Part model, mm, in its own coordinate system. A direction names the side the tool comes from. Coordinates: 2 decimals unless noted, no trailing zeros. Write each loop counter-clockwise with the first axis right and the second up, starting at its lowest first coordinate (ties: lowest second). Pieces come first, ordered by that corner, then holes. Notation, with made-up numbers: M 88,6.5 L 128,6.5 A6 cw 128,15.5 Z; hole C 10.5,-3.5 d3. An arc over 180 degrees is marked long. Use a Markdown table: item, result. Add a question column.
Q1. Slice it at D-D on x = -17.5. Write the cut outline in (y, z), then the cut area to 3 significant figures.
Q2. Slice it at B-B on z = 18.5. Write the cut outline in (x, y).
Q3. Slice it at C-C on y = 1.5. Write the cut outline in (x, z).
Q4. Slice it at A-A on x = -42. Write the cut outline in (y, z), then the cut area to 3 significant figures.
Q5. Wall check: L1, parallel to Z at x = -35.5, y = 9.75; L2, parallel to Z at x = -53.5, y = 1; L3, parallel to X at y = 1.5, z = 12. Give the ranges that are in metal, low to high. Write a range as from..to.
Q6. Tool access for faces 1 (the flat face through (-26, 23.72, 47)), 2 (the flat face through (-15, 3.72, 24)), 3 (the flat face through (-26, 17.72, 45)): list every direction of +Z, -Z, +X, -X, +Y, -Y with a clear straight run to the whole face (end or side of a thin tool).
Q7. Pin check, flat tips, straight feed: pin 1 Ø5.5 at (x, z) = (-25.82, 35.92) entering from -Y; pin 2 Ø0.5 at (x, z) = (-15, 43.5) entering from +Y; pin 3 Ø1 at (x, z) = (-23.5, 9.5) entering from +Y. Stop position of each tip, or through.
Q8. Mould opens along Y. For faces 4 (the flat face through (-44, 22.72, 1)), 5 (the conical face through (-46.144, 12.179, 5.854)), 6 (the flat face through (-26, 17.72, 3)) say: released by +Y, released by -Y, zero draft, split by the parting line, or undercut.
from build123d import *

# Parameters (mm, degrees)
SKETCH_1_W             = 25
SKETCH_1_H             = 25
EXTRUDE_1_DEPTH        = 4
SKETCH_2_W             = 24
SKETCH_2_H             = 24
EXTRUDE_2_DEPTH        = 2
SKETCH_3_R             = 5.625
EXTRUDE_3_DEPTH        = 4
CHAMFER_1_SIZE         = 3
CHAMFER_1_SIZE2        = 0.803847577
EXTRUDE_4_DEPTH        = 2
SKETCH_6_R             = 5
CUT_EXTRUDE_2_DEPTH    = 10
EXTRUDE_6_DEPTH        = 20
SKETCH_9_W             = 19
SKETCH_9_H             = 3
CUT_EXTRUDE_4_DEPTH    = 2
CHAMFER_2_SIZE         = 1
CHAMFER_3_SIZE         = 3.732050808
CHAMFER_3_SIZE_2       = 1
FILLET_1_R             = 13
CHAMFER_4_SIZE         = 1
SKETCH_11_W            = 3
SKETCH_11_H            = 4
EXTRUDE_7_DEPTH        = 16
PATTERN_LINEAR_1_COUNT = 2
PATTERN_LINEAR_1_PITCH = 22
CHAMFER_6_SIZE         = 3
FILLET_2_R             = 1.5
SKETCH_13_W            = 40.293086247
SKETCH_13_H            = 27.591529789
CUT_EXTRUDE_6_DEPTH    = 100
SKETCH_14_R            = 3
CUT_EXTRUDE_7_DEPTH    = 100
CHAMFER_7_SIZE         = 1.5


with BuildPart() as part:
    # Эскиз1 → Бобышка-Вытянуть1 (new body)
    with BuildSketch(Plane.XY):
        with Locations((-26.279531703, 11.219512195)):
            Rectangle(SKETCH_1_W, SKETCH_1_H)
    extrude(amount=EXTRUDE_1_DEPTH)

    # Эскиз2 → Бобышка-Вытянуть2 (add)
    with BuildSketch(Plane(origin=(0, 0, 0), x_dir=(-1, 0, 0), z_dir=(0, 0, -1))):
        with Locations((50.779531703, 10.719512195)):
            Rectangle(SKETCH_2_W, SKETCH_2_H)
    extrude(amount=-EXTRUDE_2_DEPTH)

    # Эскиз3 → Бобышка-Вытянуть3 (add)
    with BuildSketch(Plane.XY.offset(2)):
        with Locations((-50.779531703, 10.719512195)):
            Circle(SKETCH_3_R)
    extrude(amount=EXTRUDE_3_DEPTH)

    # Фаска1
    chamfer_1_edges = [part.edges().sort_by_distance(p)[0] for p in [
        (-56.404531703, 10.719512195, 6),
    ]]
    chamfer_1_side = [part.faces().sort_by_distance(p)[0] for p in [
        (-56.404531703, 10.719512195, 4),
    ]]
    chamfer(chamfer_1_edges, length=CHAMFER_1_SIZE, length2=CHAMFER_1_SIZE2, reference=chamfer_1_side[0])

    # Эскиз5 → Бобышка-Вытянуть4 (add)
    with BuildSketch(Plane.XY.offset(4)):
        with BuildLine():
            Line((-18.981970926, 22.719512195), (-0.779531703, 22.719512195))
            ThreePointArc((-0.779531703, 22.719512195), (11.220468297, 10.719512195), (-0.779531703, -1.280487805))
            Line((-0.779531703, -1.280487805), (-18.981970926, -1.280487805))
            ThreePointArc((-18.981970926, -1.280487805), (-30.981970926, 10.719512195), (-18.981970926, 22.719512195))
        make_face()
    extrude(amount=-EXTRUDE_4_DEPTH)

    # Эскиз6 → Вырез-Вытянуть2 (cut)
    with BuildSketch(Plane(origin=(0, 0, 2), x_dir=(-1, 0, 0), z_dir=(0, 0, -1))):
        with Locations((0.779531703, 10.719512195)):
            Circle(SKETCH_6_R)
    extrude(amount=-CUT_EXTRUDE_2_DEPTH, mode=Mode.SUBTRACT)

    # Эскиз8 → Бобышка-Вытянуть6 (add)
    with BuildSketch(Plane.XY.offset(4)):
        Polygon((-38.779531703, 3.719512195), (-35.779531703, 3.719512195), (-35.779531703, 0.719512195), (-16.779531703, 0.719512195), (-16.779531703, 3.719512195), (-13.779531703, 3.719512195), (-13.779531703, -1.280487805), (-38.779531703, -1.280487805), align=None)
    extrude(amount=EXTRUDE_6_DEPTH)

    # Эскиз9 → Вырез-Вытянуть4 (cut)
    with BuildSketch(Plane.XY.offset(4)):
        with Locations((-26.279531703, 19.219512195)):
            Rectangle(SKETCH_9_W, SKETCH_9_H)
    extrude(amount=-CUT_EXTRUDE_4_DEPTH, mode=Mode.SUBTRACT)

    # Фаска2
    chamfer_2_edges = [part.edges().sort_by_distance(p)[0] for p in [
        (-26.279531703, 20.719512195, 4),
    ]]
    chamfer(chamfer_2_edges, length=CHAMFER_2_SIZE)

    # Фаска3
    # the kernel refuses this chamfer: 3.732050808, 1 mm, written as the material it takes off along each edge
    with BuildSketch(Plane(origin=(-0.779531703, 10.719512195, 2), x_dir=(-1, 0, 0), z_dir=(0, -1, 0))) as chamfer_3_piece_1:
        Polygon((5, -CHAMFER_3_SIZE), (5 + CHAMFER_3_SIZE_2, 0), (5, 0), align=None)
    revolve(axis=Axis((-0.779531703, 10.719512195, 2), (0, 0, -1)), mode=Mode.SUBTRACT)

    # Скругление1
    fillet_1_edges = [part.edges().sort_by_distance(p)[0] for p in [
        (-62.779531703, 22.719512195, 1),
    ]]
    fillet(fillet_1_edges, radius=FILLET_1_R)

    # Фаска4
    chamfer_4_edges = [part.edges().sort_by_distance(p)[0] for p in [
        (-26.279531703, 23.719512195, 4),
    ]]
    chamfer(chamfer_4_edges, length=CHAMFER_4_SIZE)

    # Эскиз11 → Бобышка-Вытянуть7 (add)
    with BuildSketch(Plane(origin=(0, 3.719512195, 0), x_dir=(1, 0, 0), z_dir=(0, 1, 0))):
        with Locations((-37.279531703, -6)):
            Rectangle(SKETCH_11_W, SKETCH_11_H)
    extrude_7 = extrude(amount=EXTRUDE_7_DEPTH)

    # Линейный массив1: Бобышка-Вытянуть7 ×2
    with Locations(*[(i * PATTERN_LINEAR_1_PITCH, 0, 0) for i in range(1, PATTERN_LINEAR_1_COUNT)]):
        add(extrude_7)

    # Фаска6
    chamfer_6_edges = [part.edges().sort_by_distance(p)[0] for p in [
        (-37.279531703, 19.719512195, 8),
        (-15.279531703, 19.719512195, 8),
    ]]
    chamfer(chamfer_6_edges, length=CHAMFER_6_SIZE)

    # Скругление2
    fillet_2_edges = [part.edges().sort_by_distance(p)[0] for p in [
        (-37.279531703, 3.719512195, 8),
        (-15.279531703, 3.719512195, 8),
        (-15.279531703, 16.719512195, 8),
        (-37.279531703, 16.719512195, 8),
    ]]
    fillet(fillet_2_edges, radius=FILLET_2_R)

    # Эскиз13 → Вырез-Вытянуть6 (cut)
    with BuildSketch(Plane.XY.offset(4)):
        with Locations((6.36701142, 8.923747301)):
            Rectangle(SKETCH_13_W, SKETCH_13_H)
    extrude(amount=-CUT_EXTRUDE_6_DEPTH, mode=Mode.SUBTRACT)

    # Эскиз14 → Вырез-Вытянуть7 (cut)
    with BuildSketch(Plane(origin=(0, 0.719512195, 0), x_dir=(1, 0, 0), z_dir=(0, 1, 0))):
        with Locations(Location((-25.824324294, -12.079681064, 0), (0, 0, 270))):
            Circle(SKETCH_14_R)
    extrude(amount=-CUT_EXTRUDE_7_DEPTH, mode=Mode.SUBTRACT)

    # Фаска7
    chamfer_7_edges = [part.edges().sort_by_distance(p)[0] for p in [
        (-25.824324294, 0.719512195, 9.079681064),
    ]]
    chamfer(chamfer_7_edges, length=CHAMFER_7_SIZE)

    # Зеркальное отражение1: part across plane


with BuildPart() as part_1:
    add(part.part)
    add(part.part.mirror(Plane(origin=(0, 0, 24), x_dir=(1, 0, 0), z_dir=(0, 0, -1))))


solid = part_1.part
Recorded:
| question | item | result |
|---|---|---|
| 1 | outline | M -1.28,0 L 23.72,0 L 23.72,3 L 22.72,4 L 21.72,4 L 20.72,3 L 20.72,2 L 17.72,2 L 17.72,4 L 0.72,4 L 0.72,44 L 17.72,44 L 17.72,46 L 20.72,46 L 20.72,45 L 21.72,44 L 22.72,44 L 23.72,45 L 23.72,48 L -1.28,48 Z |
| 1 | area | 266 mm² |
| 2 | outline | M -38.78,-1.28 L -13.78,-1.28 L -13.78,3.72 L -16.78,3.72 L -16.78,0.72 L -35.78,0.72 L -35.78,3.72 L -38.78,3.72 Z |
| 3 | outline | M -62.78,0 L -13.78,0 L -13.78,48 L -62.78,48 L -62.78,46 L -38.78,46 L -38.78,2 L -62.78,2 Z; hole M -35.78,4 L -16.78,4 L -16.78,44 L -35.78,44 Z |
| 4 | outline | M -1.28,0 L 22.72,0 L 22.72,2 L -1.28,2 Z; M -1.28,46 L 22.72,46 L 22.72,48 L -1.28,48 Z |
| 4 | area | 96.0 mm² |
| 5 | L1 | 0..4, 44..48 |
| 5 | L2 | 0..2, 46..48 |
| 5 | L3 | -38.78..-35.78, -16.78..-13.78 |
| 6 | face 1 | +Z, -Z, +X, -X, +Y |
| 6 | face 2 | +X, -X, +Y |
| 6 | face 3 | none |
| 7 | pin 1 | through |
| 7 | pin 2 | y = 19.72 |
| 7 | pin 3 | y = 0.19 |
| 8 | face 4 | released by +Y |
| 8 | face 5 | split by the parting line |
| 8 | face 6 | undercut |
